Build history of the part. All positions in model axes, mm. A direction names the side the tool comes from. Give positions to 0.01 mm unless a question says otherwise; leave off trailing zeros. Loops run counter-clockwise (first coordinate to the right, second up) from the corner with the lowest first, then second, coordinate; pieces in that order, holes last.
1) Flat gauge pins, fed straight in: P1, Ø2, axis at x = 14, y = 4.5, coming from the -Z side; P2, Ø9, axis at x = 11, y = 15, coming from the -Z side; P3, Ø2, axis at x = 10, y = 10, coming from the +Z side. Where does each tip first touch, or does it go through?
2) Band-saw the part on B-B on y = 11.25. List the corners of the cut face in (x, z).
3) Band-saw the part on C-C on y = 8.5. List the corners of the cut face in (x, z).
4) 3-axis set-ups, long thin cutter, end or side, ignore diameter. For faces 1 (the cylindrical face through (12.73, 7.19, 6.96)), 2 (the cylindrical face through (9.75, 2.54, 2.45)), 3 (the flat face through (11, 7, 0)): which of +Z, -Z, +X, -X, +Y, -Y reach the whole face in a straight line?
5) Band-saw the part on A-A on y = 15. List the corners of the cut face in (x, z).
6) Two-plate mould, pull along X, no slides. Class faces 4 (the conical face through (4.16, 5.62, 5.35)), 5 (the flat face through (22, 13, 4)), 6 (the flat face through (0, 13, 4)), 7 (the cylindrical face through (14.06, 19.81, 2.91)): +X half, -X half, draft (parallel to the pull), parting line (faces both ways), or undercut.
7) Wall check: line 1 (X direction, y = 2.7, z = 5.5); line 2 (Z direction, x = 18, y = 3.15); line 3 (Y direction, x = 11, z = 7.2). Give the ranges that are in metal, low to high.
```python
from build123d import *

# Parameters (mm, degrees)
SKETCH1_W                       = 22
SKETCH1_H                       = 26
SKETCH1_R                       = 5.7
BOSS_EXTRUDE1_DEPTH             = 8
SKETCH3_R                       = 8
CUT_EXTRUDE2_DEPTH              = 2.1
TAP_DRILL_FOR_M3X0_5_TAP1_D     = 2.5
TAP_DRILL_FOR_M3X0_5_TAP1_DEPTH = 5
TAP_DRILL_FOR_M3X0_5_TAP1_TIP   = 0.751075774


with BuildPart() as part:
    # Sketch1 → Boss-Extrude1 (new body)
    with BuildSketch(Plane.XY):
        with Locations((11, 13)):
            Rectangle(SKETCH1_W, SKETCH1_H)
        with Locations((11, 15)):
            Circle(SKETCH1_R, mode=Mode.SUBTRACT)
    extrude(amount=BOSS_EXTRUDE1_DEPTH)

    # Sketch3 → Cut-Extrude2 (cut)
    with BuildSketch(Plane(origin=(0, 0, 8), x_dir=(-1, 0, 0), z_dir=(0, 0, -1))):
        with Locations((-11, 15)):
            Circle(SKETCH3_R)
    extrude(amount=CUT_EXTRUDE2_DEPTH, mode=Mode.SUBTRACT)

    # Tap Drill for M3x0.5 Tap1
    with Locations(Plane(origin=(0, 0, 0), x_dir=(-1, 0, 0), z_dir=(0, -1, 0))):
        with Locations((-4, -5.5), (-18, -5.5), (-11, -2.5)):
            Hole(TAP_DRILL_FOR_M3X0_5_TAP1_D / 2, depth=TAP_DRILL_FOR_M3X0_5_TAP1_DEPTH)
            with Locations((0, 0, -(TAP_DRILL_FOR_M3X0_5_TAP1_DEPTH + TAP_DRILL_FOR_M3X0_5_TAP1_TIP / 2))):  # 118° drill point
                Cone(0, TAP_DRILL_FOR_M3X0_5_TAP1_D / 2, TAP_DRILL_FOR_M3X0_5_TAP1_TIP, mode=Mode.SUBTRACT)


solid = part.part
```
Findings below:
1. P1: stops at z = 0
1. P2: passes through
1. P3: stops at z = 5.9
2. outline: (0, 0) - (6.71, 0) - (6.71, 5.9) - (3.93, 5.9) - (3.93, 8) - (0, 8) - close; (15.29, 0) - (22, 0) - (22, 8) - (18.07, 8) - (18.07, 5.9) - (15.29, 5.9) - close
3. outline: (0, 0) - (22, 0) - (22, 8) - (15.66, 8) - (15.66, 5.9) - (6.34, 5.9) - (6.34, 8) - (0, 8) - close
4. face 1: +Z
4. face 2: -Y
4. face 3: -Z, +X, -X, +Y, -Y
5. outline: (0, 0) - (5.3, 0) - (5.3, 5.9) - (3, 5.9) - (3, 8) - (0, 8) - close; (16.7, 0) - (22, 0) - (22, 8) - (19, 8) - (19, 5.9) - (16.7, 5.9) - close
6. face 4: undercut
6. face 5: +X half
6. face 6: -X half
6. face 7: undercut
7. line 1: x = 0 to 2.75, 5.25 to 16.75, 19.25 to 22
7. line 2: z = 0 to 4.25, 6.75 to 8
7. line 3: y = 0 to 7, 23 to 26
